```python
from build123d import *

# Parameters (mm, degrees)
SKETCH_1_R          = 10.75
EXTRUDE_1_DEPTH     = 1.35
SKETCH_4_R          = 9.25
EXTRUDE_3_DEPTH     = 7.3
EXTRUDE_START       = 8.65
SKETCH_1_4_R        = 10.75
EXTRUDE_4_DEPTH     = 1.35
SKETCH_6_R          = 7.5
EXTRUDE_5_DEPTH     = 7
SKETCH_5_R          = 4
CUT_EXTRUDE_1_DEPTH = 23.806249144


with BuildPart() as part:
    # 草图1 → 凸台-拉伸1 (new body)
    with BuildSketch(Plane(origin=(0, 0, 0), x_dir=(1, 0, 0), z_dir=(0, 1, 0))):
        with Locations(Location((0, 0, 0), (0, 0, 90))):
            Circle(SKETCH_1_R)
    extrude(amount=EXTRUDE_1_DEPTH)

    # 草图4 → 凸台-拉伸3 (add)
    with BuildSketch(Plane(origin=(0, 1.35, 0), x_dir=(1, 0, 0), z_dir=(0, 1, 0))):
        with Locations(Location((0, 0, 0), (0, 0, 270))):
            Circle(SKETCH_4_R)
    extrude(amount=EXTRUDE_3_DEPTH)

    # 草图1<4> → 凸台-拉伸4 (add)
    with BuildSketch(Plane(origin=(0, 0, 0), x_dir=(1, 0, 0), z_dir=(0, 1, 0)).offset(EXTRUDE_START)):
        with Locations(Location((0, 0, 0), (0, 0, 90))):
            Circle(SKETCH_1_4_R)
    extrude(amount=EXTRUDE_4_DEPTH)

    # 草图6 → 凸台-拉伸5 (add)
    with BuildSketch(Plane(origin=(0, 10, 0), x_dir=(1, 0, 0), z_dir=(0, 1, 0))):
        with Locations(Location((0, 0, 0), (0, 0, 270))):
            Circle(SKETCH_6_R)
    extrude(amount=EXTRUDE_5_DEPTH)

    # 草图5 → 切除-拉伸1 (cut, through all)
    with BuildSketch(Plane.XZ):
        with Locations(Location((0, 0, 0), (0, 0, 270))):
            Circle(SKETCH_5_R)
    extrude(amount=-CUT_EXTRUDE_1_DEPTH, mode=Mode.SUBTRACT)


solid = part.part
```
The listing builds one solid part. Answer for the finished solid, in the listing's coordinates (mm). A direction names the side the tool comes from. Give positions to 0.01 mm unless a question says otherwise; leave off trailing zeros. Order: outer loops, then holes, each group sorted by start corner. A loop starts at its lowest first (then second) coordinate and runs counter-clockwise, first axis right, second up. Notation, with made-up numbers: M -16.75,66.25 L -11.75,66.25 A30 cw -11.75,90.25 Z; hole C -36.5,-5.5 d10. An arc over 180 degrees is marked long. Put each result on its own line as item: value. Start each with the question number.
Item 1: The part is cut by section D-D, the plane x = 4.75. Determine the outline of the cut face in (y, z), and give its area (3 significant figures).
Item 2: The part is cut by section A-A, the plane x = 0. Determine the outline of the cut face in (y, z).
Item 3: Which of the six approach directions +Z, -Z, +X, -X, +Y, -Y give full straight-line access (tool end or side, diameter ignored) to faces 4 (the face through (-7.32, 10, -2.24)), 5 (the face through (-3, 17, 3)), 6 (the face through (-3.543, 4.949, 8.545))?
Item 4: For a pull along Z with two mould halves and no side action, classify faces 1 (the face through (-8, 1.35, -5)), 2 (the face through (-7.27, 0.67, 7.92)), 3 (the face through (-3.905, 8.381, 0.867)) as +Z half, -Z half, draft (parallel to the pull), parting line (faces both ways), or undercut.
Item 5: Flat-ended cylindrical pins translate along their axes: P1, Ø2, axis at y = 13, z = 2.5, coming from the +X side; P2, Ø1.5, axis at y = 2, z = 6, coming from the -X side; P3, Ø2, axis at y = 3, z = 2.5, coming from the +X side; P4, Ø1, axis at x = 1.5, z = -1.5, coming from the +Y side. Find the tip coordinate at first contact, or state that the pin passes through.
Item 6: The part is cut by section B-B, the plane z = 0. Determine the outline of the cut face in (x, y).
Item 7: Find the intervals of material crossed by line 1 along X through (y, z) = (4, 0); line 2 along Y through (x, z) = (-5.25, 8.5); line 3 along X through (y, z) = (13.25, 0), in increasing order.
Item 8: The part is cut by section C-C, the plane y = 5.75. Determine the outline of the cut face in (x, z), and give its area (3 significant figures).
Answer key:
1. outline: M 0,-9.64 L 1.35,-9.64 L 1.35,-7.94 L 8.65,-7.94 L 8.65,-9.64 L 10,-9.64 L 10,-5.8 L 17,-5.8 L 17,5.8 L 10,5.8 L 10,9.64 L 8.65,9.64 L 8.65,7.94 L 1.35,7.94 L 1.35,9.64 L 0,9.64 Z
1. area: 249 mm²
2. outline: M 0,-10.75 L 1.35,-10.75 L 1.35,-9.25 L 8.65,-9.25 L 8.65,-10.75 L 10,-10.75 L 10,-7.5 L 17,-7.5 L 17,-4 L 0,-4 Z; M 0,4 L 17,4 L 17,7.5 L 10,7.5 L 10,10.75 L 8.65,10.75 L 8.65,9.25 L 1.35,9.25 L 1.35,10.75 L 0,10.75 Z
3. face 4: +Y
3. face 5: +Z, -Z, +X, -X, +Y
3. face 6: none
4. face 1: draft
4. face 2: parting line
4. face 3: undercut
5. P1: stops at x = 7.35
5. P2: stops at x = -9.16
5. P3: stops at x = 9.13
5. P4: passes through
6. outline: M -10.75,0 L -4,0 L -4,17 L -7.5,17 L -7.5,10 L -10.75,10 L -10.75,8.65 L -9.25,8.65 L -9.25,1.35 L -10.75,1.35 Z; M 4,0 L 10.75,0 L 10.75,1.35 L 9.25,1.35 L 9.25,8.65 L 10.75,8.65 L 10.75,10 L 7.5,10 L 7.5,17 L 4,17 Z
7. line 1: x = -9.25 to -4, 4 to 9.25
7. line 2: y = 0 to 1.35, 8.65 to 10
7. line 3: x = -7.5 to -4, 4 to 7.5
8. outline: C 0,0 d18.5; hole C 0,0 d8
8. area: 219 mm²
